```python
from build123d import *

# Parameters (mm, degrees)
F1_DEPTH = 25
F2_DEPTH = 8


with BuildPart() as f1:
    # F0 (on Top) → F1 (new body)
    with BuildSketch(Plane.XY):
        with BuildLine():
            ThreePointArc((0, -4), (2.828427, -2.828427), (4, 0))
            ThreePointArc((4, 0), (2.828427, 2.828427), (0, 4))
            Line((0, 4), (0, 2.5))
            ThreePointArc((0, 2.5), (1.767767, 1.767767), (2.5, 0))
            ThreePointArc((2.5, 0), (1.767767, -1.767767), (0, -2.5))
            Line((0, -2.5), (0, -4))
        make_face()
        with BuildLine():
            Line((0, 2.5), (0, 4))
            ThreePointArc((0, 4), (-2.828427, 2.828427), (-4, 0))
            ThreePointArc((-4, 0), (-2.828427, -2.828427), (0, -4))
            Line((0, -4), (0, -2.5))
            ThreePointArc((0, -2.5), (-2.5, 0), (0, 2.5))
        make_face()
        with BuildLine():
            Line((-4, -4), (0, -4))
            ThreePointArc((0, -4), (-2.828427, -2.828427), (-4, 0))
            Line((-4, 0), (-4, -4))
        make_face()
        with BuildLine():
            ThreePointArc((-4, 0), (-2.828427, 2.828427), (0, 4))
            Line((0, 4), (-4, 4))
            Line((-4, 4), (-4, 0))
        make_face()
        with BuildLine():
            ThreePointArc((2.5, 0), (1.767767, 1.767767), (0, 2.5))
            Line((0, 2.5), (0, -2.5))
            ThreePointArc((0, -2.5), (1.767767, -1.767767), (2.5, 0))
        make_face()
        with BuildLine():
            Line((0, -2.5), (0, 2.5))
            ThreePointArc((0, 2.5), (-2.5, 0), (0, -2.5))
        make_face()
    extrude(amount=-F1_DEPTH)

    # F0 (on Top) → F2 (join)
    with BuildSketch(Plane.XY):
        with BuildLine():
            Line((0, -2.5), (0, 2.5))
            ThreePointArc((0, 2.5), (-2.5, 0), (0, -2.5))
        make_face()
        with BuildLine():
            ThreePointArc((2.5, 0), (1.767767, 1.767767), (0, 2.5))
            Line((0, 2.5), (0, -2.5))
            ThreePointArc((0, -2.5), (1.767767, -1.767767), (2.5, 0))
        make_face()
    extrude(amount=F2_DEPTH)


solid = f1.part
```
Geometry check sheet. Reference: the model listing, model coordinates, mm. A direction names the side the tool comes from. Give positions to 0.01 mm unless a question says otherwise; leave off trailing zeros. Order: outer loops, then holes, each group sorted by start corner. A loop starts at its lowest first (then second) coordinate and runs counter-clockwise, first axis right, second up.
1. Section check C-C, the plane z = -2.5. Enter the section's corners in (x, y), and give its area (3 significant figures).
2. Thickness scan on L1, parallel to X at y = 0, z = 3.5; L2, parallel to Z at x = 0.5, y = 3.75; L3, parallel to X at y = 2, z = -4.5. Record the ranges inside material, lowest first.
3. Access from +Z, -Z, +X, -X, +Y, -Y to the whole of each face (thin tool, end or side, straight path). Record for faces 1 (the face through (-2, -2, 0)), 2 (the face through (-2, 4, -12)).
4. Gauge pin test, flat end, axial feed: pin 1 Ø1 at (x, z) = (1.5, -7) entering from +Y. Record the tip position at first contact, or that the pin passes through.
5. Section check B-B, the plane x = -1.75. Enter the section's corners in (y, z).
6. Section check A-A, the plane y = -1.5. Enter the section's corners in (x, z).
7. Section check D-D, the plane y = -3. Enter the section's corners in (x, z), and give its area (3 significant figures).
Values follow:
1. outline: (-4, -4) - (0, -4) arc R4 ccw to (0, 4) - (-4, 4) - close
1. area: 57.1 mm2
2. L1: x = -2.5 to 2.5
2. L2: z = -25 to 0
2. L3: x = -4 to 3.46
3. face 1: +Z
3. face 2: +Z, -Z, +X, -X, +Y
4. pin 1: stops at y = 3.87
5. outline: (-4, -25) - (4, -25) - (4, 0) - (1.79, 0) - (1.79, 8) - (-1.79, 8) - (-1.79, 0) - (-4, 0) - close
6. outline: (-4, -25) - (3.71, -25) - (3.71, 0) - (2, 0) - (2, 8) - (-2, 8) - (-2, 0) - (-4, 0) - close
7. outline: (-4, -25) - (2.65, -25) - (2.65, 0) - (-4, 0) - close
7. area: 166 mm2
